Model file for the job. Use its own axes, mm. Give positions to 0.01 mm unless a question says otherwise; leave off trailing zeros. Write each loop counter-clockwise with the first axis right and the second up, starting at its lowest first coordinate (ties: lowest second). Pieces come first, ordered by that corner, then holes. Notation, with made-up numbers: (77, 22) - (107, 22) arc R23 cw to (107, 51) - close; hole circle Ø2 at (-17.5, 37). An arc over 180 degrees is marked (long way). Use CSV: the item, a comma, the result in double quotes.
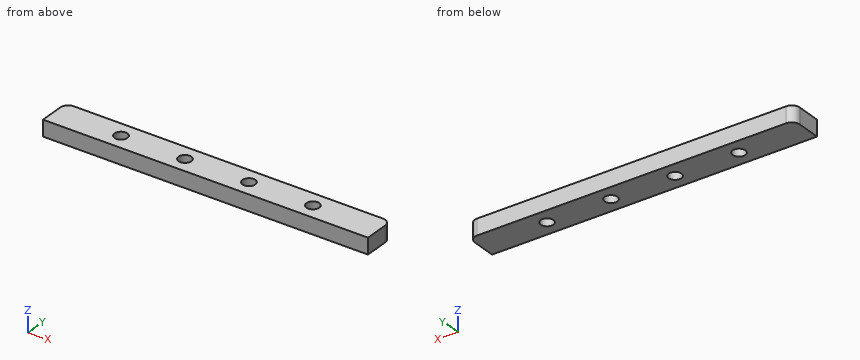
from build123d import *

# Parameters (mm, degrees)
SKETCH1_W           = 101.6
SKETCH1_H           = 10
BOSS_EXTRUDE1_DEPTH = 5
SKETCH2_R           = 2
CUT_EXTRUDE1_DEPTH  = 5
FILLET1_R           = 2.5


with BuildPart() as part:
    # Sketch1 → Boss-Extrude1 (new body)
    with BuildSketch(Plane.XY):
        with Locations((0, 5)):
            Rectangle(SKETCH1_W, SKETCH1_H)
    extrude(amount=BOSS_EXTRUDE1_DEPTH)

    # Sketch2 → Cut-Extrude1 (cut)
    with BuildSketch(Plane.XY.offset(5)):
        with Locations((-30, 5)):
            Circle(SKETCH2_R)
        with Locations((-10, 5)):
            Circle(SKETCH2_R)
        with Locations((10, 5)):
            Circle(SKETCH2_R)
        with Locations((30, 5)):
            Circle(SKETCH2_R)
    extrude(amount=-CUT_EXTRUDE1_DEPTH, mode=Mode.SUBTRACT)

    # Fillet1
    fillet1_edges = [part.edges().sort_by_distance(p)[0] for p in [
        (-50.8, 10, 2.5),
        (50.8, 10, 2.5),
    ]]
    fillet(fillet1_edges, radius=FILLET1_R)


solid = part.part
(1) Saw through at C-C, the plane z = 1.15. List the corners of the cut face in (x, y).
Checked values:
outline,"(-50.8, 0) - (50.8, 0) - (50.8, 7.5) arc R2.5 ccw to (48.3, 10) - (-48.3, 10) arc R2.5 ccw to (-50.8, 7.5) - close; hole circle Ø4 at (-30, 5); hole circle Ø4 at (-10, 5); hole circle Ø4 at (10, 5); hole circle Ø4 at (30, 5)"
(2) Wall check: probe 1 along X at (y, z) = (6.5, 1.35); probe 2 along Y at (x, z) = (-10, 4); probe 3 along X at (y, z) = (4, 1.75). Give the ranges that are in metal, low to high. Write a range as [from, to].
Checked values:
probe 1,"x = [-50.8, -31.32], [-28.68, -11.32], [-8.68, 8.68], [11.32, 28.68], [31.32, 50.8]"
probe 2,"y = [0, 3], [7, 10]"
probe 3,"x = [-50.8, -31.73], [-28.27, -11.73], [-8.27, 8.27], [11.73, 28.27], [31.73, 50.8]"
(3) Flat gauge pin, fed straight in: P1, Ø1.5, axis at x = 7.5, y = 2.5, coming from the -Z side. Where does the tip first touch, or does it go through?
Checked values:
P1,"stops at z = 0"
(4) Saw through at D-D, the plane x = 31. List the corners of the cut face in (y, z).
Checked values:
outline,"(0, 0) - (3.27, 0) - (3.27, 5) - (0, 5) - close; (6.73, 0) - (10, 0) - (10, 5) - (6.73, 5) - close"
(5) Saw through at A-A, the plane y = 5. List the corners of the cut face in (x, z), then the cut area to 3 significant figures.
Checked values:
outline,"(-50.8, 0) - (-32, 0) - (-32, 5) - (-50.8, 5) - close; (-28, 0) - (-12, 0) - (-12, 5) - (-28, 5) - close; (-8, 0) - (8, 0) - (8, 5) - (-8, 5) - close; (12, 0) - (28, 0) - (28, 5) - (12, 5) - close; (32, 0) - (50.8, 0) - (50.8, 5) - (32, 5) - close"
area,"428 mm^2"
(6) Saw through at B-B, the plane x = 10. List the corners of the cut face in (y, z), then the cut area to 3 significant figures.
Checked values:
outline,"(0, 0) - (3, 0) - (3, 5) - (0, 5) - close; (7, 0) - (10, 0) - (10, 5) - (7, 5) - close"
area,"30.0 mm^2"
